For this review, take the finished solid that the model builds, in its own axes (mm). Face numbers are marked on the shaded views. A direction names the side the tool comes from. Give positions to 0.01 mm unless a question says otherwise; leave off trailing zeros. Loops run counter-clockwise (first coordinate to the right, second up) from the corner with the lowest first, then second, coordinate; pieces in that order, holes last. Notation, with made-up numbers: (-38, -18) - (-29, -18) arc R37 ccw to (-29, 21) - close; hole circle Ø3 at (5, 42.5). An arc over 180 degrees is marked (long way). Answer as CSV lines item,"result".
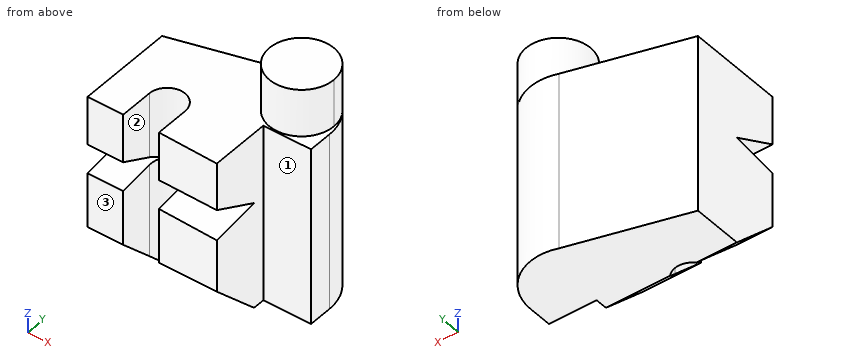
from build123d import *

# Parameters (mm, degrees)
F1_DEPTH = 75
F3_DEPTH = 75
F5_DEPTH = 75
F7_DEPTH = 20


with BuildPart() as f1:
    # F0 (on Top) → F1 (new body)
    with BuildSketch(Plane.XY):
        with BuildLine():
            Line((-37.5, 20.907951), (-37.5, -19.092049))
            Line((-37.5, -19.092049), (-22.5, -19.092049))
            Line((-22.5, -19.092049), (-22.5, -5.092049))
            ThreePointArc((-22.5, -5.092049), (-15, 2.407951), (-7.5, -5.092049))
            Line((-7.5, -5.092049), (-7.5, -19.092049))
            Line((-7.5, -19.092049), (17.483507, -20))
            Line((17.483507, -20), (17.483507, 5))
            Line((17.483507, 5), (37.483507, 5))
            Line((37.483507, 5), (37.483507, 15))
            ThreePointArc((37.483507, 15), (29.021611, 31.336222), (10.796291, 33.848903))
            Line((10.796291, 33.848903), (-37.5, 20.907951))
        make_face()
    extrude(amount=F1_DEPTH)

    # F2 (on face) → F3 (cut)
    with BuildSketch(Plane.YZ.offset(17.483507)):
        Polygon((-20, 42.03419), (0, 45), (-20, 55), align=None)
    extrude(amount=-F3_DEPTH, mode=Mode.SUBTRACT)

    # F4 (on face) → F5 (cut)
    with BuildSketch(Plane.YZ.offset(17.483507)):
        Polygon((-20, 20), (-20, 0), (0, 0), align=None)
    extrude(amount=-F5_DEPTH, mode=Mode.SUBTRACT)

    # F6 (on face) → F7 (join)
    with BuildSketch(Plane.XY.offset(75)):
        with BuildLine():
            ThreePointArc((33.248047, 27.307692), (9.84171, 14.607072), (36.106982, 19))
            ThreePointArc((36.106982, 19), (35.372255, 23.392928), (33.248047, 27.307692))
        make_face()
    extrude(amount=F7_DEPTH)


solid = f1.part
1) Consider section A-A on y = -3. Write out the cut boundary in (x, z).
From the geometry:
outline,"(-37.5, 3) - (-22.2, 3) - (-22.2, 44.56) - (-37.5, 44.56) - close; (-37.5, 46.5) - (-22.2, 46.5) - (-22.2, 75) - (-37.5, 75) - close; (-7.8, 3) - (17.48, 3) - (17.48, 44.56) - (-7.8, 44.56) - close; (-7.8, 46.5) - (17.48, 46.5) - (17.48, 75) - (-7.8, 75) - close"
2) Consider section C-C on x = 13. Write out the cut boundary in (y, z), and give its area (3 significant figures).
From the geometry:
outline,"(-19.84, 19.84) - (0, 0) - (34.49, 0) - (34.49, 75) - (28.48, 75) - (28.48, 95) - (9.52, 95) - (9.52, 75) - (-19.84, 75) - (-19.84, 54.92) - (0, 45) - (-19.84, 42.06) - close"
area,"4,130 mm^2"
3) Insertion check: P1, Ø4.5, axis at x = -29.5, z = 68.5, coming from the -Y side; P2, Ø15.5, axis at y = -11.5, z = 24, coming from the +X side; P3, Ø10, axis at x = 23.5, z = 43, coming from the -Y side; P4, Ø5, axis at x = -18.5, y = -10.5, coming from the +Z side. Each pin has a flat end and moves straight along its axis. Give the tip position at first contact, or say it passes through.
From the geometry:
P1,"stops at y = -19.09"
P2,"stops at x = 17.48"
P3,"stops at y = 5"
P4,"passes through"
4) Consider section D-D on y = -14.5. Write out the cut boundary in (x, z).
From the geometry:
outline,"(-37.5, 14.5) - (-22.5, 14.5) - (-22.5, 42.85) - (-37.5, 42.85) - close; (-37.5, 52.25) - (-22.5, 52.25) - (-22.5, 75) - (-37.5, 75) - close; (-7.5, 14.5) - (17.48, 14.5) - (17.48, 42.85) - (-7.5, 42.85) - close; (-7.5, 52.25) - (17.48, 52.25) - (17.48, 75) - (-7.5, 75) - close"
5) Consider section B-B on z = 16.5. Write out the cut boundary in (x, y), and give its area (3 significant figures).
From the geometry:
outline,"(-37.5, -16.5) - (-22.5, -16.5) - (-22.5, -5.09) arc R7.5 cw to (-7.5, -5.09) - (-7.5, -16.5) - (17.48, -16.5) - (17.48, 5) - (37.48, 5) - (37.48, 15) arc R20 ccw to (10.8, 33.85) - (-37.5, 20.91) - close"
area,"2,720 mm^2"
6) Wall thickness on line 1 (X direction, y = -16.5, z = 26); line 2 (Z direction, x = 6, y = 19.5); line 3 (Z direction, x = 9, y = -1): over which ranges is each line inside the solid? List them lowest first. Write a range as from..to.
From the geometry:
line 1,"x = -37.5..-22.5, -7.5..17.48"
line 2,"z = 0..75"
line 3,"z = 1..44.85, 45.5..75"
7) Machinability: for the marked faces 1, 2 and 3, which of the approach directions +Z, -Z, +X, -X, +Y, -Y give a long, thin tool a straight path to every point of the face, cutting with its end or side? Answer none if there is none.
From the geometry:
face 1,"+Z, -Z, +X, -Y"
face 2,"+Z, -Z, -Y"
face 3,"+Z, -Z, -X, -Y"
